from build123d import *

# Parameters (mm, degrees)
SKIZZE1_W                       = 55.85
SKIZZE1_H                       = 2
AUFSATZ_LINEAR_AUSTRAGEN1_DEPTH = 5
SKIZZE2_W                       = 4
SKIZZE2_H                       = 11.6
AUFSATZ_LINEAR_AUSTRAGEN2_DEPTH = 5
LINEARES_MUSTER1_COUNT          = 11
LINEARES_MUSTER1_PITCH          = 5.185
AUFSATZ_LINEAR_AUSTRAGEN3_DEPTH = 1
LINEARES_MUSTER2_COUNT          = 10
LINEARES_MUSTER2_PITCH          = 5.185
LINEARES_MUSTER2_COPY_1_DEPTH   = 1
LINEARES_MUSTER2_COPY_2_DEPTH   = 1
LINEARES_MUSTER2_COPY_3_DEPTH   = 1
LINEARES_MUSTER2_COPY_4_DEPTH   = 1
LINEARES_MUSTER2_COPY_5_DEPTH   = 1
LINEARES_MUSTER2_COPY_6_DEPTH   = 1
LINEARES_MUSTER2_COPY_7_DEPTH   = 1
LINEARES_MUSTER2_COPY_8_DEPTH   = 1
LINEARES_MUSTER2_COPY_9_DEPTH   = 1


with BuildPart() as part:
    # Skizze1 → Aufsatz-Linear austragen1 (new, symmetric)
    with BuildSketch(Plane.XY):
        with Locations((27.925, -1)):
            Rectangle(SKIZZE1_W, SKIZZE1_H)
    extrude(amount=AUFSATZ_LINEAR_AUSTRAGEN1_DEPTH, both=True)

    # Skizze2 → Aufsatz-Linear austragen2 (add, symmetric)
    with BuildSketch(Plane.XY):
        with Locations((2, 5.8)):
            Rectangle(SKIZZE2_W, SKIZZE2_H)
    aufsatz_linear_austragen2 = extrude(amount=AUFSATZ_LINEAR_AUSTRAGEN2_DEPTH, both=True)

    # Lineares Muster1: Aufsatz-Linear austragen2 ×11
    with Locations(*[(i * LINEARES_MUSTER1_PITCH, 0, 0) for i in range(1, LINEARES_MUSTER1_COUNT)]):
        add(aufsatz_linear_austragen2)

    # Skizze3 → Aufsatz-Linear austragen3 (add)
    with BuildSketch(Plane.XY.offset(5)):
        with BuildLine():
            Line((4, 8.6), (4, 0))
            Line((4, 0), (5.185, 0))
            Line((5.185, 0), (5.185, 8.6))
            ThreePointArc((5.185, 8.6), (4.5925, 8.0075), (4, 8.6))
        make_face()
    aufsatz_linear_austragen3 = extrude(amount=-AUFSATZ_LINEAR_AUSTRAGEN3_DEPTH)

    # Spiegeln1: Aufsatz-Linear austragen3 across plane
    add(aufsatz_linear_austragen3.mirror(Plane.XY))

    # Lineares Muster2: Aufsatz-Linear austragen3 ×10
    with Locations(*[(i * LINEARES_MUSTER2_PITCH, 0, 0) for i in range(1, LINEARES_MUSTER2_COUNT)]):
        add(aufsatz_linear_austragen3)

    # Lineares Muster2 copy 1 sketch → Lineares Muster2 copy 1 (add)
    with BuildSketch(Plane(origin=(5.185, 0, -5), x_dir=(1, 0, 0), z_dir=(0, 0, -1))):
        with BuildLine():
            Line((4, -8.6), (4, 0))
            Line((4, 0), (5.185, 0))
            Line((5.185, 0), (5.185, -8.6))
            ThreePointArc((5.185, -8.6), (4.5925, -8.0075), (4, -8.6))
        make_face()
    extrude(amount=-LINEARES_MUSTER2_COPY_1_DEPTH)

    # Lineares Muster2 copy 2 sketch → Lineares Muster2 copy 2 (add)
    with BuildSketch(Plane(origin=(10.37, 0, -5), x_dir=(1, 0, 0), z_dir=(0, 0, -1))):
        with BuildLine():
            Line((4, -8.6), (4, 0))
            Line((4, 0), (5.185, 0))
            Line((5.185, 0), (5.185, -8.6))
            ThreePointArc((5.185, -8.6), (4.5925, -8.0075), (4, -8.6))
        make_face()
    extrude(amount=-LINEARES_MUSTER2_COPY_2_DEPTH)

    # Lineares Muster2 copy 3 sketch → Lineares Muster2 copy 3 (add)
    with BuildSketch(Plane(origin=(15.555, 0, -5), x_dir=(1, 0, 0), z_dir=(0, 0, -1))):
        with BuildLine():
            Line((4, -8.6), (4, 0))
            Line((4, 0), (5.185, 0))
            Line((5.185, 0), (5.185, -8.6))
            ThreePointArc((5.185, -8.6), (4.5925, -8.0075), (4, -8.6))
        make_face()
    extrude(amount=-LINEARES_MUSTER2_COPY_3_DEPTH)

    # Lineares Muster2 copy 4 sketch → Lineares Muster2 copy 4 (add)
    with BuildSketch(Plane(origin=(20.74, 0, -5), x_dir=(1, 0, 0), z_dir=(0, 0, -1))):
        with BuildLine():
            Line((4, -8.6), (4, 0))
            Line((4, 0), (5.185, 0))
            Line((5.185, 0), (5.185, -8.6))
            ThreePointArc((5.185, -8.6), (4.5925, -8.0075), (4, -8.6))
        make_face()
    extrude(amount=-LINEARES_MUSTER2_COPY_4_DEPTH)

    # Lineares Muster2 copy 5 sketch → Lineares Muster2 copy 5 (add)
    with BuildSketch(Plane(origin=(25.925, 0, -5), x_dir=(1, 0, 0), z_dir=(0, 0, -1))):
        with BuildLine():
            Line((4, -8.6), (4, 0))
            Line((4, 0), (5.185, 0))
            Line((5.185, 0), (5.185, -8.6))
            ThreePointArc((5.185, -8.6), (4.5925, -8.0075), (4, -8.6))
        make_face()
    extrude(amount=-LINEARES_MUSTER2_COPY_5_DEPTH)

    # Lineares Muster2 copy 6 sketch → Lineares Muster2 copy 6 (add)
    with BuildSketch(Plane(origin=(31.11, 0, -5), x_dir=(1, 0, 0), z_dir=(0, 0, -1))):
        with BuildLine():
            Line((4, -8.6), (4, 0))
            Line((4, 0), (5.185, 0))
            Line((5.185, 0), (5.185, -8.6))
            ThreePointArc((5.185, -8.6), (4.5925, -8.0075), (4, -8.6))
        make_face()
    extrude(amount=-LINEARES_MUSTER2_COPY_6_DEPTH)

    # Lineares Muster2 copy 7 sketch → Lineares Muster2 copy 7 (add)
    with BuildSketch(Plane(origin=(36.295, 0, -5), x_dir=(1, 0, 0), z_dir=(0, 0, -1))):
        with BuildLine():
            Line((4, -8.6), (4, 0))
            Line((4, 0), (5.185, 0))
            Line((5.185, 0), (5.185, -8.6))
            ThreePointArc((5.185, -8.6), (4.5925, -8.0075), (4, -8.6))
        make_face()
    extrude(amount=-LINEARES_MUSTER2_COPY_7_DEPTH)

    # Lineares Muster2 copy 8 sketch → Lineares Muster2 copy 8 (add)
    with BuildSketch(Plane(origin=(41.48, 0, -5), x_dir=(1, 0, 0), z_dir=(0, 0, -1))):
        with BuildLine():
            Line((4, -8.6), (4, 0))
            Line((4, 0), (5.185, 0))
            Line((5.185, 0), (5.185, -8.6))
            ThreePointArc((5.185, -8.6), (4.5925, -8.0075), (4, -8.6))
        make_face()
    extrude(amount=-LINEARES_MUSTER2_COPY_8_DEPTH)

    # Lineares Muster2 copy 9 sketch → Lineares Muster2 copy 9 (add)
    with BuildSketch(Plane(origin=(46.665, 0, -5), x_dir=(1, 0, 0), z_dir=(0, 0, -1))):
        with BuildLine():
            Line((4, -8.6), (4, 0))
            Line((4, 0), (5.185, 0))
            Line((5.185, 0), (5.185, -8.6))
            ThreePointArc((5.185, -8.6), (4.5925, -8.0075), (4, -8.6))
        make_face()
    extrude(amount=-LINEARES_MUSTER2_COPY_9_DEPTH)


solid = part.part
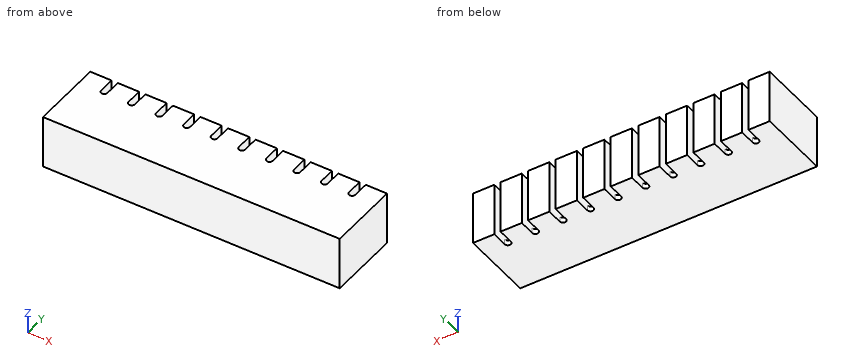
Check sheet for the modelled part. Datum: model origin and axes. Units: mm. Give positions to 0.01 mm unless a question says otherwise; leave off trailing zeros. Use one line per item in the form item = value. Start each with the question number.
1. Thickness scan on line 1 along Z through (x, y) = (25, 6.5); line 2 along Y through (x, z) = (15, -3.75); line 3 along Y through (x, z) = (40.5, 4.5). Record the ranges inside material, lowest first. Write a range as from..to.
2. Go/stop test with a flat-tipped pin: P1, Ø3, axis at y = 8, z = 2, coming from the -X side. Record where the tip stops, or that it passes through.
3. Section check A-A (y = 1.75). Count the separate pieces of the cut face and the enclosed holes in it, and give its area (3 significant figures).
Conclusion:
q1.line_1 = -5..-4, 4..5
q1.line_2 = -2..0
q1.line_3 = -2..8.15
q2.P1 = 0
q3.separate_pieces = 1
q3.enclosed_holes = 10
q3.area = 464 mm²
